Drawing for the job (mm, zero at the part's lowest x, y, z). Round coordinates to 2 decimals unless told otherwise and drop trailing zeros. Write each loop counter-clockwise with the first axis right and the second up, starting at its lowest first coordinate (ties: lowest second). Pieces come first, ordered by that corner, then holes. Notation, with made-up numbers: (-33, 85.5) - (22, 85.5) arc R32 cw to (22, 114.5) - close; hole circle Ø3 at (79, 67). An arc over 180 degrees is marked (long way). Answer in a Markdown table with one row per item.
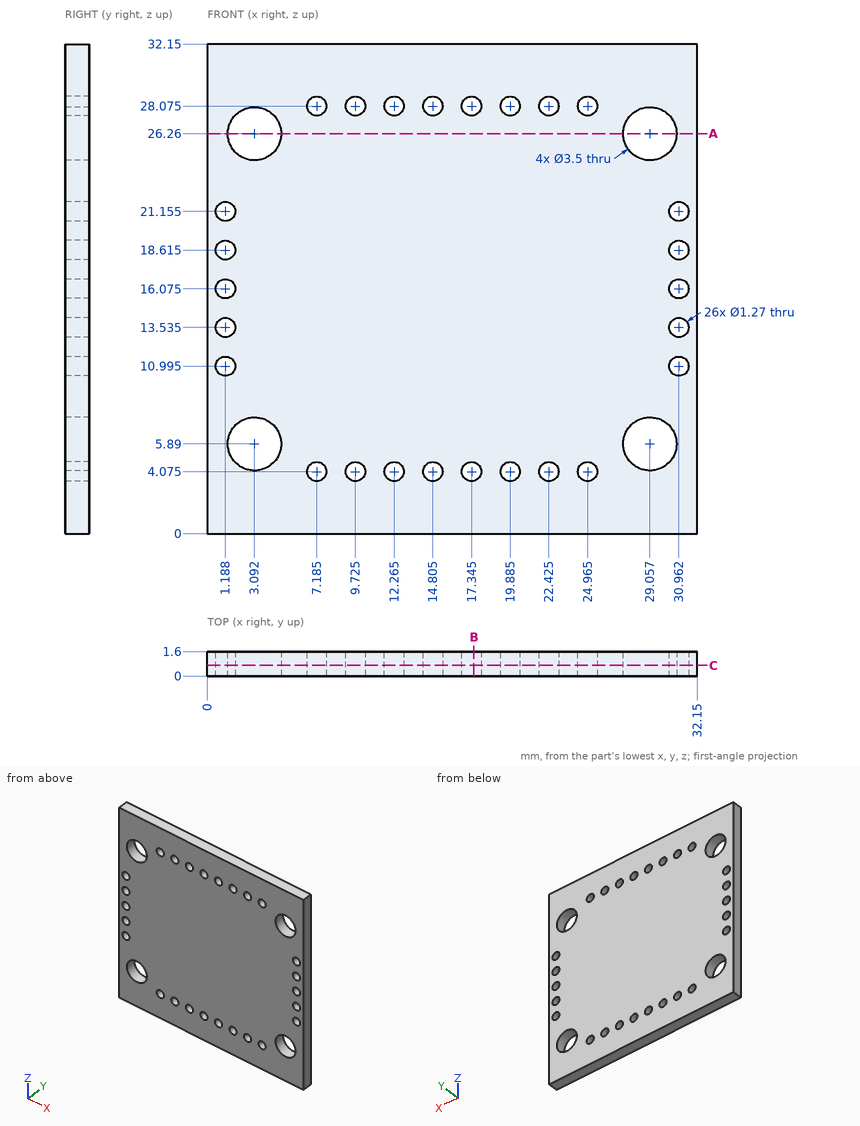
Q1. Saw through at C-C on y = 0.7. Count the separate pieces of the cut face and the enclosed holes in it, then the cut area to 3 significant figures.
Computed:
| item | result |
|---|---|
| separate pieces | 1 |
| enclosed holes | 30 |
| area | 962 mm2 |
Q2. Flat gauge pins, fed straight in: pin 1 (3 mm diameter, centred on x = 3.09, z = 26.26, fed in from +Y); pin 2 (1.5 mm diameter, centred on x = 22.425, z = 4.075, fed in from -Y). Where does each tip first touch, or does it go through?
Computed:
| item | result |
|---|---|
| pin 1 | passes through |
| pin 2 | stops at y = 0 |
Q3. Saw through at B-B on x = 17.5. List the corners of the cut face in (y, z).
Computed:
| item | result |
|---|---|
| outline | (0, 0) - (1.6, 0) - (1.6, 3.46) - (0, 3.46) - close; (0, 4.69) - (1.6, 4.69) - (1.6, 27.46) - (0, 27.46) - close; (0, 28.69) - (1.6, 28.69) - (1.6, 32.15) - (0, 32.15) - close |
Q4. Drill centre lines: line 1 (Z direction, x = 25, y = 1.55); line 2 (Z direction, x = 3, y = 1.4); line 3 (X direction, y = 0.65, z = 18.5). Where is each one in solid material? Low to high.
Computed:
| item | result |
|---|---|
| line 1 | z = 0 to 3.44, 4.71 to 27.44, 28.71 to 32.15 |
| line 2 | z = 0 to 4.14, 7.64 to 24.51, 28.01 to 32.15 |
| line 3 | x = 0 to 0.56, 1.81 to 30.34, 31.59 to 32.15 |
Q5. Saw through at A-A on z = 26.26. List the corners of the cut face in (x, y).
Computed:
| item | result |
|---|---|
| outline | (0, 0) - (1.34, 0) - (1.34, 1.6) - (0, 1.6) - close; (4.84, 0) - (27.31, 0) - (27.31, 1.6) - (4.84, 1.6) - close; (30.81, 0) - (32.15, 0) - (32.15, 1.6) - (30.81, 1.6) - close |
